```python
from build123d import *

# Parameters (mm, degrees)
SKETCH1_R           = 3.81
BOSS_EXTRUDE1_DEPTH = 12.7
SKETCH5_W           = 108.117548543
SKETCH5_H           = 153.094987558
CUT_EXTRUDE2_DEPTH  = 18.78
FILLET1_R           = 6.35
CUT_EXTRUDE3_DEPTH  = 13.7
SKETCH4_R           = 4.7625
CUT_EXTRUDE1_DEPTH  = 12.7


with BuildPart() as part:
    # Sketch1 → Boss-Extrude1 (new body)
    with BuildSketch(Plane.XY):
        with BuildLine():
            Line((0, 25.4), (0, 0))
            Line((0, 0), (27.038931816, 0))
            ThreePointArc((27.038931816, 0), (25.425, 12.7), (27.038931816, 25.4))
            Line((27.038931816, 25.4), (0, 25.4))
        make_face()
        with Locations((12.7, 12.7)):
            Circle(SKETCH1_R, mode=Mode.SUBTRACT)
        with BuildLine():
            ThreePointArc((27.038931816, 25.4), (25.425, 12.7), (27.038931816, 0))
            Line((27.038931816, 0), (40.305493108, 0))
            ThreePointArc((40.305493108, 0), (38.125, 12.7), (40.305493108, 25.4))
            Line((40.305493108, 25.4), (27.038931816, 25.4))
        make_face()
        with BuildLine():
            ThreePointArc((69.85, 63.076364746), (42.655301643, 50.816319827), (27.038931816, 25.4))
            Line((27.038931816, 25.4), (40.305493108, 25.4))
            ThreePointArc((40.305493108, 25.4), (51.696372754, 41.842372532), (69.85, 50.241751757))
            Line((69.85, 50.241751757), (69.85, 63.076364746))
        make_face()
        with BuildLine():
            Line((40.305493108, 0), (27.038931816, 0))
            ThreePointArc((27.038931816, 0), (42.655301643, -25.416319827), (69.85, -37.676364746))
            Line((69.85, -37.676364746), (69.85, -24.841751757))
            ThreePointArc((69.85, -24.841751757), (51.696372754, -16.442372532), (40.305493108, 0))
        make_face()
    extrude(amount=BOSS_EXTRUDE1_DEPTH)

    # Sketch5 → Cut-Extrude2 (cut, through all)
    with BuildSketch(Plane(origin=(52.07, 0, 0), x_dir=(0, 0, -1), z_dir=(1, 0, 0))):
        with Locations((4.394422663, 1.362842318)):
            Rectangle(SKETCH5_W, SKETCH5_H)
    extrude(amount=CUT_EXTRUDE2_DEPTH, mode=Mode.SUBTRACT)

    # Fillet1
    fillet1_edges = [part.edges().sort_by_distance(p)[0] for p in [
        (52.07, 57.374866816, 6.35),
        (52.07, -31.974866816, 6.35),
    ]]
    fillet(fillet1_edges, radius=FILLET1_R)

    # Sketch6 → Cut-Extrude3 (cut, through all)
    with BuildSketch(Plane.XY.offset(12.7)):
        with BuildLine():
            Line((9.525, 16.51), (15.875, 16.51))
            ThreePointArc((15.875, 16.51), (19.685, 12.7), (15.875, 8.89))
            Line((15.875, 8.89), (9.525, 8.89))
            ThreePointArc((9.525, 8.89), (5.715, 12.7), (9.525, 16.51))
        make_face()
    extrude(amount=-CUT_EXTRUDE3_DEPTH, mode=Mode.SUBTRACT)

    # Sketch4 → Cut-Extrude1 (cut)
    with BuildSketch(Plane(origin=(53.975, 0, 0), x_dir=(0, 0, -1), z_dir=(1, 0, 0))):
        with Locations((-6.35, -31.259058251)):
            Circle(SKETCH4_R)
        with Locations((-6.35, 56.659058251)):
            Circle(SKETCH4_R)
    extrude(amount=-CUT_EXTRUDE1_DEPTH, mode=Mode.SUBTRACT)


solid = part.part
```
Here's how the part is built. I have some questions about the finished solid (model axes, mm). A direction names the side the tool comes from. Give positions to 0.01 mm unless a question says otherwise; leave off trailing zeros. Loops run counter-clockwise (first coordinate to the right, second up) from the corner with the lowest first, then second, coordinate; pieces in that order, holes last. Notation, with made-up numbers: M 29.25,44 L 34.25,44 A21 ccw 34.25,70 Z; hole C 32.25,77.5 d1. An arc over 180 degrees is marked long. Put each result on its own line as item: value. Start each with the question number.
(1) I need wall thicknesses on line 1 along Y through (x, z) = (5.5, 8.75); line 2 along X through (y, z) = (11.5, 8.5); line 3 along X through (y, z) = (10.5, 3). Which ranges of each line are inside material? Lowest first, please. Write a range as [from, to].
(2) I want a section at B-B on x = 39. Please give me the cut outline in (y, z).
(3) If we mould it in two halves opening along Y, with no side actions, what happens to faces 4 (the flat face through (13, 0, 6)), 5 (the flat face through (52.07, -18, 6)), 6 (the flat face through (13, 16.51, 6))? For each: +Y half, -Y half, draft (parallel to the pull), parting line (faces both ways), or undercut.
(4) I want a section at A-A on y = 12.7. Please give me the cut outline in (x, z) (3 decimals), then the cut area to 3 significant figures.
(5) I want a section at D-D on x = 24.5. Please give me the cut outline in (y, z).
(6) For faces 1 (the flat face through (13, 8.89, 6)), 2 (the flat face through (14, 25.4, 6)), 3 (the cylindrical face through (48.14, 50.89, 6.26)), which set-ups out of +Z, -Z, +X, -X, +Y, -Y let a thin tool reach every point of the face, with its end or its side?
(7) Will these pins go through, and if not, where does the flat tip stop? pin 1 Ø2 at (y, z) = (33.5, 8) entering from -X; pin 2 Ø6 at (y, z) = (-13.5, 5.5) entering from +X; pin 3 Ø10 at (x, y) = (29, 42.5) entering from +Z; pin 4 Ø5 at (x, z) = (11.5, 6.5) entering from +Y.
Answer block:
1. line 1: [0, 25.4]
1. line 2: [0, 5.91], [19.49, 38.14]
1. line 3: [0, 6.41], [18.99, 38.19]
2. outline: M -21.86,0 L 4.58,0 L 4.58,12.7 L -21.86,12.7 Z; M 20.82,0 L 47.26,0 L 47.26,12.7 L 20.82,12.7 Z
3. face 4: -Y half
3. face 5: draft
3. face 6: undercut
4. outline: M 0,0 L 5.715,0 L 5.715,12.7 L 0,12.7 Z; M 19.685,0 L 38.125,0 L 38.125,12.7 L 19.685,12.7 Z
4. area: 307 mm^2
5. outline: M 0,0 L 25.4,0 L 25.4,12.7 L 0,12.7 Z
6. face 1: +Z, -Z
6. face 2: +Z, -Z, -X, +Y
6. face 3: +Z, -Z, +Y
7. pin 1: x = 29.44
7. pin 2: x = 51.77
7. pin 3: through
7. pin 4: y = 25.4
